Check sheet for the modelled part. Datum: model origin and axes. Units: mm. A direction names the side the tool comes from. Give positions to 0.01 mm unless a question says otherwise; leave off trailing zeros. Loops run counter-clockwise (first coordinate to the right, second up) from the corner with the lowest first, then second, coordinate; pieces in that order, holes last. Notation, with made-up numbers: M 49.5,56 L 94.5,56 A11 cw 94.5,61 Z; hole C -19,85.5 d1. An arc over 180 degrees is marked long. Use one line per item in the form item = value.
from build123d import *

# Parameters (mm, degrees)
F0_R     = 40
F1_DEPTH = 10
F2_R     = 30
F3_DEPTH = 10
F4_R     = 20
F5_DEPTH = 150
F6_R     = 7.5
F7_DEPTH = 15
F8_SIZE2 = 9.99999
F8_SIZE  = 9.99999
F9_SIZE  = 9.99999
F10_SIZE = 3


# Not quite as in the source:
# - a fillet or chamfer is up to 0.001 mm smaller than in the source, because OpenCascade refuses the exact size


with BuildPart() as f1:
    # F0 (on Top) → F1 (new body)
    with BuildSketch(Plane.XY):
        Circle(F0_R)
    extrude(amount=F1_DEPTH)

    # F2 (on Top) → F3 (join)
    with BuildSketch(Plane.XY):
        Circle(F2_R)
    extrude(amount=-F3_DEPTH)

    # F4 (on face) → F5 (join)
    with BuildSketch(Plane(origin=(0, 0, -10), x_dir=(1, 0, 0), z_dir=(0, 0, -1))):
        Circle(F4_R)
    extrude(amount=F5_DEPTH)

    # F6 (on face) → F7 (join)
    with BuildSketch(Plane(origin=(0, 0, -160), x_dir=(1, 0, 0), z_dir=(0, 0, -1))):
        Circle(F6_R)
    extrude(amount=F7_DEPTH)

    # F8 (size 10 and 10 in the source; OpenCascade refuses exactly that, so slightly less here)
    f8_edges = [f1.edges().sort_by_distance(p)[0] for p in [
        (-40, 0, 10),
    ]]
    chamfer(f8_edges, length=F8_SIZE, length2=F8_SIZE2)

    # F9 (size 10 in the source; OpenCascade refuses exactly that, so slightly less here)
    f9_edges = [f1.edges().sort_by_distance(p)[0] for p in [
        (-30, 0, -10),
    ]]
    chamfer(f9_edges, length=F9_SIZE)

    # F10
    f10_edges = [f1.edges().sort_by_distance(p)[0] for p in [
        (-20, 0, -160),
    ]]
    chamfer(f10_edges, length=F10_SIZE)


solid = f1.part
1) Depth check by flat-ended pin: pin 1 Ø3 at (x, y) = (20, -4.5) entering from -Z; pin 2 Ø1.5 at (x, y) = (1.5, -21) entering from -Z; pin 3 Ø3 at (x, z) = (-18.5, -49) entering from -Y. Enter the tip coordinate at first touch or a pass-through.
Evaluation:
pin_1 = -158
pin_2 = -9.7
pin_3 = -10.54
2) Set-up check for faces 1 (the face through (0, 0, -175)), 2 (the face through (-4.336, 19.524, -82.471)): record each of +Z, -Z, +X, -X, +Y, -Y from which the full face is reachable in a straight line by a thin tool's end or side.
Evaluation:
face_1 = -Z, +X, -X, +Y, -Y
face_2 = -Z
3) Section check C-C (z = -28.5). Record the cut outline in (x, y), then the cut area to 3 significant figures.
Evaluation:
outline = C 0,0 d40
area = 1,260 mm^2
4) Scan lines: line 1 (Z direction, x = 3, y = -15.5); line 2 (Y direction, x = -7, z = -137) (3 decimals); line 3 (Y direction, x = -0.5, z = -13.5). Record each from-to range of solid material in increasing order.
Evaluation:
line_1 = -160 to 10
line_2 = -18.735 to 18.735
line_3 = -19.99 to 19.99
